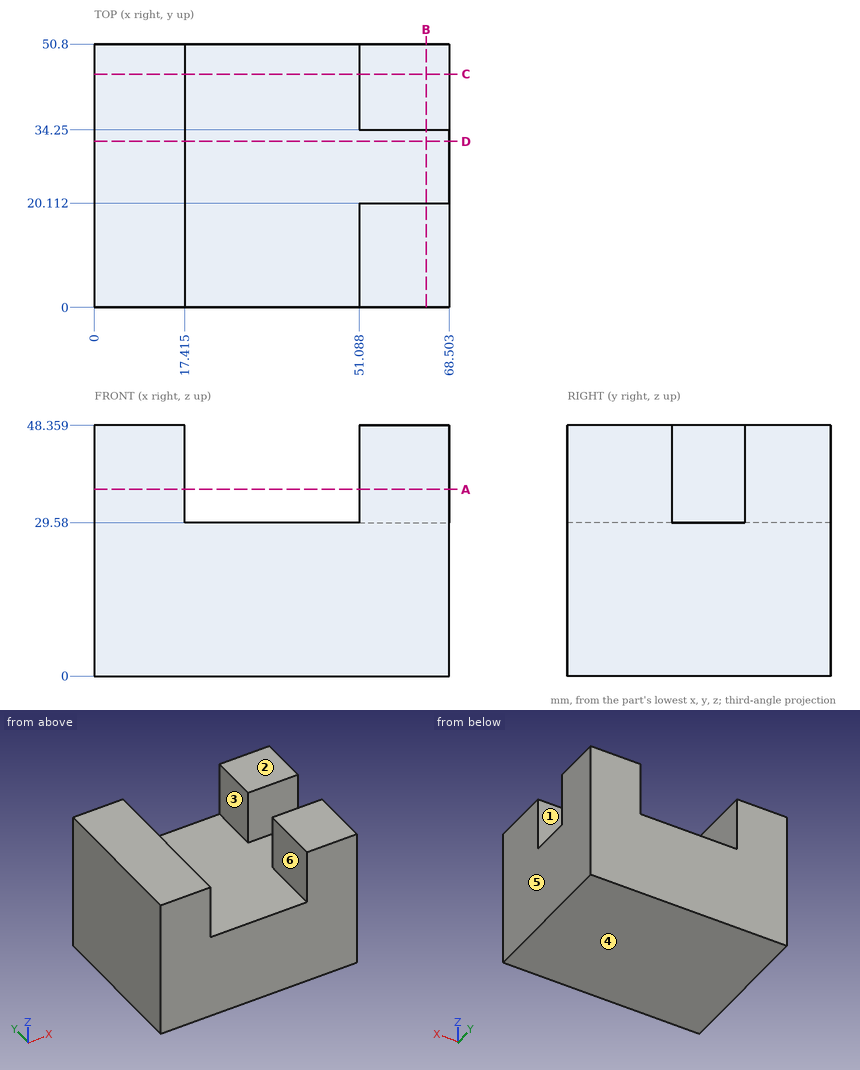
Input: dimensioned drawing with shaded views. Units: mm. Origin: part minimum x, y, z. A direction names the side the tool comes from. Give positions to 0.01 mm unless a question says otherwise; leave off trailing zeros. Loops run counter-clockwise (first coordinate to the right, second up) from the corner with the lowest first, then second, coordinate; pieces in that order, holes last. Notation, with made-up numbers: (1, 12) -> (40, 12) arc R26 ccw to (40, 30) -> close; hole circle Ø7 at (50, -15.5). An arc over 180 degrees is marked (long way). Use a Markdown table: item, result. Add a question column.
1) Reachability of the marked faces 1, 2 and 3 from +Z, -Z, +X, -X, +Y, -Y: full face, straight path, thin tool, end or side. Return the list, or none.
2) Section query A-A, the plane z = 36. Count the separate pieces of the cut face and the enclosed holes in it, then the cut area to 3 significant figures.
3) Line query: line 1 along X through (y, z) = (9, 46) (1 decimal); line 2 along X through (y, z) = (32, 45.5) (1 decimal); line 3 along Z through (x, y) = (25, 6.5). Output: solid intervals per line, ascending. Write a range as [from, to].
4) Section query C-C, the plane y = 45. Return the cut outline in (x, z) (1 decimal).
5) Pull-direction query (X, two-part tool) for the marked faces 4, 5 and 6; classes: +X half, -X half, draft (parallel to the pull), parting line (faces both ways), or undercut.
6) Section query B-B, the plane x = 64. Return the cut outline in (y, z), then the cut area to 3 significant figures.
7) Section query D-D, the plane y = 32. Return the cut outline in (x, z) (1 decimal), then the cut area to 3 significant figures.
Numbers:
| question | item | result |
|---|---|---|
| 1 | face 1 | +Z, +X |
| 1 | face 2 | +Z, +X, -X, +Y, -Y |
| 1 | face 3 | +Z, +Y, -Y |
| 2 | separate pieces | 3 |
| 2 | enclosed holes | 0 |
| 2 | area | 1,520 mm2 |
| 3 | line 1 | x = [0, 17.4], [51.1, 68.5] |
| 3 | line 2 | x = [0, 17.4] |
| 3 | line 3 | z = [0, 29.58] |
| 4 | outline | (0, 0) -> (68.5, 0) -> (68.5, 48.4) -> (51.1, 48.4) -> (51.1, 29.6) -> (17.4, 29.6) -> (17.4, 48.4) -> (0, 48.4) -> close |
| 5 | face 4 | draft |
| 5 | face 5 | +X half |
| 5 | face 6 | undercut |
| 6 | outline | (0, 0) -> (50.8, 0) -> (50.8, 48.36) -> (34.25, 48.36) -> (34.25, 29.58) -> (20.11, 29.58) -> (20.11, 48.36) -> (0, 48.36) -> close |
| 6 | area | 2,190 mm2 |
| 7 | outline | (0, 0) -> (68.5, 0) -> (68.5, 29.6) -> (17.4, 29.6) -> (17.4, 48.4) -> (0, 48.4) -> close |
| 7 | area | 2,350 mm2 |
